Could you check a few things on this drawing? It's one solid part, dimensions in mm from its lowest x, y, z. A direction names the side the tool comes from. Give positions to 0.01 mm unless a question says otherwise; leave off trailing zeros. Loops run counter-clockwise (first coordinate to the right, second up) from the corner with the lowest first, then second, coordinate; pieces in that order, holes last. Notation, with made-up numbers: (69.5, -15) - (100.5, -15) arc R16 ccw to (100.5, 7) - close; hole circle Ø2 at (8, 32). An arc over 180 degrees is marked (long way). Answer as a JSON object with one key per item and string values.
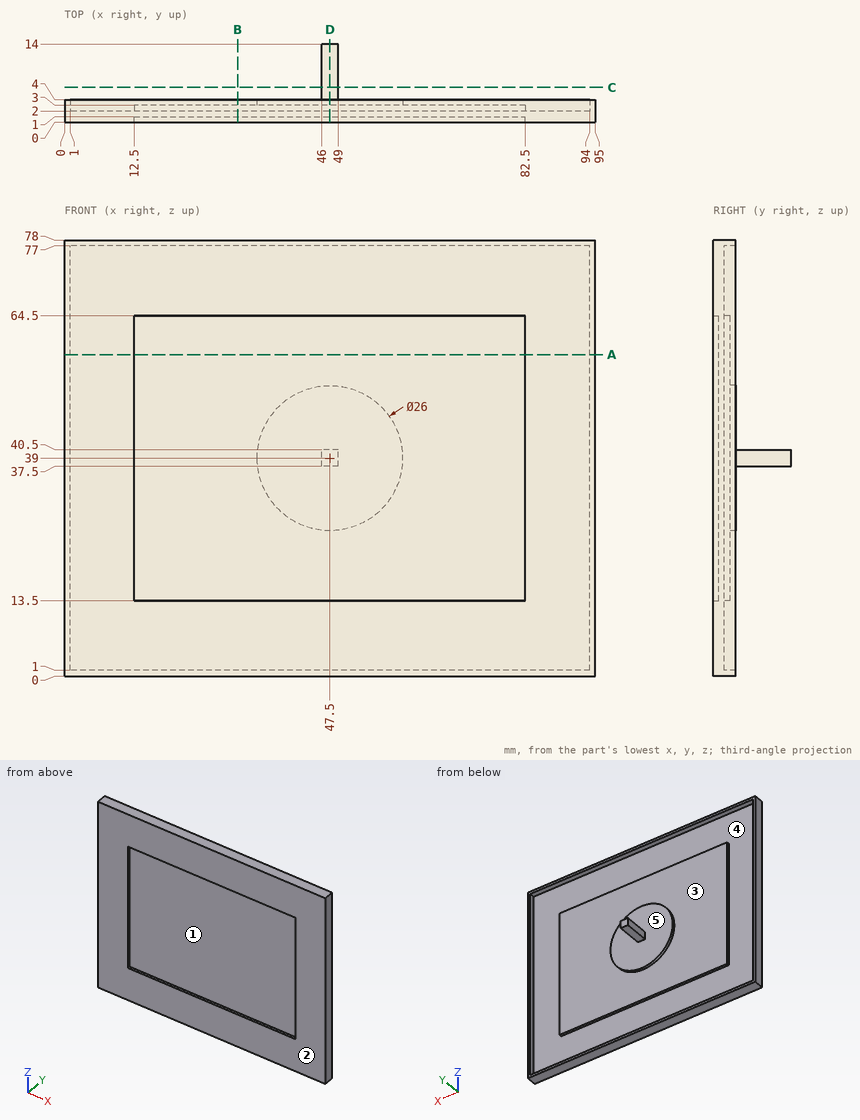
1) If we mould it in two halves opening along X, with no side actions, what happens to the marked faces 4 and 5? For each: released by +X, released by -X, zero draft, split by the parting line, or undercut.
Check sheet entries:
{"face 4": "undercut", "face 5": "zero draft"}
2) Imagine slicing it at B-B on x = 31. Write out the boundary of the cut face in (y, z).
Check sheet entries:
{"outline": "(0, 0) - (4, 0) - (4, 1) - (2, 1) - (2, 13.5) - (3, 13.5) - (3, 64.5) - (2, 64.5) - (2, 77) - (4, 77) - (4, 78) - (0, 78) - (0, 64.5) - (1, 64.5) - (1, 13.5) - (0, 13.5) - close"}
3) Which directions (+Z, -Z, +X, -X, +Y, -Y) give clear straight access to the entire face, cutting with the end or side of a thin tool? Please do the marked faces 1, 2 and 3.
Check sheet entries:
{"face 1": "-Y", "face 2": "+Z, -Z, +X, -X, -Y", "face 3": "+Y"}
4) I'm going to push flat-ended pins straight in: P1, Ø2.5, axis at x = 47.5, y = 11, coming from the -Z side; P2, Ø1.5, axis at x = 47.5, y = 9, coming from the +Z side; P3, Ø3.5, axis at y = 6.5, z = 39.5, coming from the -X side. Where does each tip first touch, or does it pass through?
Check sheet entries:
{"P1": "z = 37.5", "P2": "z = 40.5", "P3": "x = 46"}
5) I need wall thicknesses on L1, parallel to X at y = 2.75, z = 53.5; L2, parallel to X at y = 3.5, z = 71; L3, parallel to Z at x = 24.5, y = 2.75. Which ranges of each line are inside material? Lowest first, please.
Check sheet entries:
{"L1": "0 to 1, 12.5 to 82.5, 94 to 95", "L2": "0 to 1, 94 to 95", "L3": "0 to 1, 13.5 to 64.5, 77 to 78"}
6) Imagine slicing it at D-D on x = 47.5. Write out the boundary of the cut face in (y, z), and give its area (3 significant figures).
Check sheet entries:
{"outline": "(0, 0) - (4, 0) - (4, 1) - (2, 1) - (2, 13.5) - (3, 13.5) - (3, 26) - (4, 26) - (4, 37.5) - (14, 37.5) - (14, 40.5) - (4, 40.5) - (4, 52) - (3, 52) - (3, 64.5) - (2, 64.5) - (2, 77) - (4, 77) - (4, 78) - (0, 78) - (0, 64.5) - (1, 64.5) - (1, 13.5) - (0, 13.5) - close", "area": "216 mm2"}
7) Imagine slicing it at C-C on y = 6.25. Write out the boundary of the cut face in (x, z), and give its area (3 significant figures).
Check sheet entries:
{"outline": "(46, 37.5) - (49, 37.5) - (49, 40.5) - (46, 40.5) - close", "area": "9.00 mm2"}
8) Imagine slicing it at A-A on z = 57.5. Write out the boundary of the cut face in (x, y), and give its area (3 significant figures).
Check sheet entries:
{"outline": "(0, 0) - (12.5, 0) - (12.5, 1) - (82.5, 1) - (82.5, 0) - (95, 0) - (95, 4) - (94, 4) - (94, 2) - (82.5, 2) - (82.5, 3) - (12.5, 3) - (12.5, 2) - (1, 2) - (1, 4) - (0, 4) - close", "area": "194 mm2"}
